Here's how the part is built. I have some questions about the finished solid (model axes, mm). A direction names the side the tool comes from. Coordinates: 2 decimals unless noted, no trailing zeros. Order: outer loops, then holes, each group sorted by start corner. A loop starts at its lowest first (then second) coordinate and runs counter-clockwise, first axis right, second up. Notation, with made-up numbers: (69.25, 13) - (102.25, 13) arc R14 ccw to (102.25, 40) - close; hole circle Ø7 at (-36.5, -19.5). An arc over 180 degrees is marked (long way). Answer in a Markdown table with one row per item. Add a question column.
Item 1: Thinking about a two-plate mould opening in Y: for faces 1 (the flat face through (21.89, 6.92, 1.48)), 2 (the cylindrical face through (-13.36, -4.18, 1.48)), 3 (the cylindrical face through (-12.176, 6.913, 1.479)), which applies, +Y half, -Y half, draft (parallel to the pull), parting line (faces both ways), or undercut?
Item 2: I want a section at B-B (x = 7.5). Please give me the cut outline in (y, z), plus the area to 3 significant figures.
Item 3: I want a section at A-A (x = 30.73). Please give me the cut outline in (y, z).
Item 4: If I drill on line 1 along Y through (x, z) = (0, 1.65); line 2 along X through (y, z) = (13.25, 2.1); line 3 along Y through (x, z) = (-7.5, 0.6), over which ranges is the centre line in solid material (lowest first)? Write a range as from..to.
Item 5: I want a section at D-D (z = 1.15). Count the separate pieces of the cut face and the enclosed holes in it, plus the area to 3 significant figures.
Item 6: I want a section at C-C (y = -8.5). Please give me the cut outline in (x, z), plus the area to 3 significant figures.
Item 7: On a 3-axis mill with a long thin cutter (end or side, diameter ignored), from which of +Z, -Z, +X, -X, +Y, -Y can I reach the whole of each face in a straight line? I mean faces 4 (the cylindrical face through (-8.66, 11.04, 1.48)), 5 (the flat face through (22.351, -1.088, 1.479)), 6 (the cylindrical face through (-12.776, 2.118, 1.479)), 7 (the cylindrical face through (12.67, 5.96, 1.48)). Say none if no direction works.
Item 8: Will these pins go through, and if not, where does the flat tip stop? pin 1 Ø3.5 at (x, y) = (30.73, 4.05) entering from +Z; pin 2 Ø1.5 at (x, z) = (-7, 2.5) entering from -Y.
```python
from build123d import *

# Parameters (mm, degrees)
SKETCH1_R           = 1.5
BOSS_EXTRUDE1_DEPTH = 3


with BuildPart() as part:
    # Sketch1 → Boss-Extrude1 (new body)
    with BuildSketch(Plane.XY):
        with BuildLine():
            Line((31.252104769, 0.084220555), (13.197893843, -2.292661406))
            ThreePointArc((13.197893843, -2.292661406), (12.969095602, -2.316113876), (12.73932764, -2.326377285))
            ThreePointArc((12.73932764, -2.326377285), (0.959824701, -12.914380997), (-12.255459075, -4.184043841))
            ThreePointArc((-12.255459075, -4.184043841), (-13.378578492, -4.178547185), (-14.474839872, -3.934337388))
            Line((-14.474839872, -3.934337388), (-14.625059689, -3.332810991))
            ThreePointArc((-14.625059689, -3.332810991), (-13.772322314, -2.601875695), (-12.783651334, -2.068999412))
            ThreePointArc((-12.783651334, -2.068999412), (-12.874361077, -1.397614704), (-12.929834926, -0.722404858))
            ThreePointArc((-12.929834926, -0.722404858), (-14.009823049, -0.414098041), (-14.999545068, 0.116823575))
            Line((-14.999545068, 0.116823575), (-14.981904447, 0.736572564))
            ThreePointArc((-14.981904447, 0.736572564), (-13.963584904, 1.210337006), (-12.867808226, 1.456712552))
            ThreePointArc((-12.867808226, 1.456712552), (-12.774016779, 2.12767369), (-12.645264071, 2.792811588))
            ThreePointArc((-12.645264071, 2.792811588), (-13.60202312, 3.381062861), (-14.411802625, 4.159320268))
            Line((-14.411802625, 4.159320268), (-14.22760989, 4.7513279))
            ThreePointArc((-14.22760989, 4.7513279), (-13.119232281, 4.932784547), (-11.997618648, 4.87438681))
            ThreePointArc((-11.997618648, 4.87438681), (-11.726282094, 5.495162259), (-11.422851828, 6.100897975))
            ThreePointArc((-11.422851828, 6.100897975), (-12.185423363, 6.925465798), (-12.755202711, 7.893339205))
            Line((-12.755202711, 7.893339205), (-12.418118595, 8.413698983))
            ThreePointArc((-12.418118595, 8.413698983), (-11.301886217, 8.289390025), (-10.23762058, 7.930550098))
            ThreePointArc((-10.23762058, 7.930550098), (-9.80886271, 8.455099783), (-9.353258921, 8.95650867))
            ThreePointArc((-9.353258921, 8.95650867), (-9.865086498, 9.956238618), (-10.152607763, 11.041945282))
            Line((-10.152607763, 11.041945282), (-9.687632252, 11.452064502))
            ThreePointArc((-9.687632252, 11.452064502), (-8.646330954, 11.031209366), (-7.718345028, 10.398540764))
            ThreePointArc((-7.718345028, 10.398540764), (-7.163964851, 10.787961235), (-6.589977589, 11.147856089))
            ThreePointArc((-6.589977589, 11.147856089), (-6.813101299, 12.248602767), (-6.797040342, 13.371620791))
            Line((-6.797040342, 13.371620791), (-6.238658543, 13.641082786))
            ThreePointArc((-6.238658543, 13.641082786), (-5.349516879, 12.954894372), (-4.626635134, 12.095319232))
            ThreePointArc((-4.626635134, 12.095319232), (-3.987748493, 12.320728954), (-3.337947765, 12.51241802))
            ThreePointArc((-3.337947765, 12.51241802), (-3.255819543, 13.632544082), (-2.937367534, 14.709584358))
            Line((-2.937367534, 14.709584358), (-2.32699207, 14.818404364))
            ThreePointArc((-2.32699207, 14.818404364), (-1.65595361, 13.917774128), (-1.191788878, 12.895043205))
            ThreePointArc((-1.191788878, 12.895043205), (-0.515779071, 12.93972457), (0.161642374, 12.948991148))
            ThreePointArc((0.161642374, 12.948991148), (0.542931453, 14.005421967), (1.140156387, 14.956605344))
            Line((1.140156387, 14.956605344), (1.757256759, 14.89671268))
            ThreePointArc((1.757256759, 14.89671268), (2.160424164, 13.848436246), (2.331446907, 12.738400815))
            ThreePointArc((2.331446907, 12.738400815), (2.994443325, 12.59904001), (3.649244238, 12.425196839))
            ThreePointArc((3.649244238, 12.425196839), (4.301415708, 13.339581776), (5.133120125, 14.094363334))
            Line((5.133120125, 14.094363334), (5.711177894, 13.870199965))
            ThreePointArc((5.711177894, 13.870199965), (5.81657316, 12.752023201), (5.681769941, 11.63700951))
            ThreePointArc((5.681769941, 11.63700951), (6.282581558, 11.323942289), (6.86619835, 10.979882523))
            ThreePointArc((6.86619835, 10.979882523), (7.740883637, 11.684405828), (8.745383825, 12.186806873))
            Line((8.745383825, 12.186806873), (9.241527091, 11.81499797))
            ThreePointArc((9.241527091, 11.81499797), (9.041333534, 10.709850931), (8.610702091, 9.672554446))
            ThreePointArc((8.610702091, 9.672554446), (9.104769458, 9.208999572), (9.573917942, 8.720240549))
            ThreePointArc((9.573917942, 8.720240549), (10.606245638, 9.162650954), (11.709042415, 9.375410697))
            Line((11.709042415, 9.375410697), (12.086474501, 8.883531626))
            ThreePointArc((12.086474501, 8.883531626), (11.595539562, 7.873378012), (10.901017858, 6.990730267))
            ThreePointArc((10.901017858, 6.990730267), (11.251698258, 6.411067486), (11.571583838, 5.813858226))
            ThreePointArc((11.571583838, 5.813858226), (12.684990922, 5.961344174), (13.804294894, 5.868683199))
            Line((13.804294894, 5.868683199), (13.809047255, 5.856830152))
            Line((13.809047255, 5.856830152), (30.207895231, 8.015779445))
            ThreePointArc((30.207895231, 8.015779445), (34.695779445, 4.572104769), (31.252104769, 0.084220555))
        make_face()
        Circle(SKETCH1_R, mode=Mode.SUBTRACT)
        with Locations((7.5, 0)):
            Circle(SKETCH1_R, mode=Mode.SUBTRACT)
        with Locations((-7.5, 0)):
            Circle(SKETCH1_R, mode=Mode.SUBTRACT)
        with Locations((30.73, 4.05)):
            Circle(SKETCH1_R, mode=Mode.SUBTRACT)
    extrude(amount=BOSS_EXTRUDE1_DEPTH)


solid = part.part
```
Values follow:
| question | item | result |
|---|---|---|
| 1 | face 1 | +Y half |
| 1 | face 2 | -Y half |
| 1 | face 3 | undercut |
| 2 | outline | (-10.56, 0) - (-1.5, 0) - (-1.5, 3) - (-10.56, 3) - close; (1.5, 0) - (11.52, 0) - (11.52, 3) - (1.5, 3) - close |
| 2 | area | 57.2 mm^2 |
| 3 | outline | (0.02, 0) - (2.55, 0) - (2.55, 3) - (0.02, 3) - close; (5.55, 0) - (8.05, 0) - (8.05, 3) - (5.55, 3) - close |
| 4 | line 1 | y = -12.95..-1.5, 1.5..12.95 |
| 4 | line 2 | x = -6.81..-5.68, -3.31..-1.32, 0.24..2.28, 4.22..5.8 |
| 4 | line 3 | y = -10.56..-1.5, 1.5..10.56 |
| 5 | separate pieces | 1 |
| 5 | enclosed holes | 4 |
| 5 | area | 706 mm^2 |
| 6 | outline | (-9.77, 0) - (9.77, 0) - (9.77, 3) - (-9.77, 3) - close |
| 6 | area | 58.6 mm^2 |
| 7 | face 4 | +Z, -Z, +Y |
| 7 | face 5 | +Z, -Z, +X, -Y |
| 7 | face 6 | +Z, -Z, -X |
| 7 | face 7 | +Z, -Z |
| 8 | pin 1 | stops at z = 3 |
| 8 | pin 2 | stops at y = -11.34 |
